Check sheet for the modelled part. Datum: model origin and axes. Units: mm. A direction names the side the tool comes from. Round coordinates to 2 decimals unless told otherwise and drop trailing zeros. Loops run counter-clockwise (first coordinate to the right, second up) from the corner with the lowest first, then second, coordinate; pieces in that order, holes last. Notation, with made-up numbers: (18, 17) - (29, 17) arc R17 cw to (29, 45) - close; hole circle Ø10 at (48, -29.5). An arc over 180 degrees is marked (long way). Put each result on its own line as item: value.
```python
from build123d import *

# Parameters (mm, degrees)
SKETCH1_W           = 44
SKETCH1_H           = 25
SKETCH1_R           = 8.5
SKETCH1_W_2         = 7.5
SKETCH1_H_2         = 4
BOSS_EXTRUDE1_DEPTH = 4
CHAMFER1_SIZE       = 4


with BuildPart() as part:
    # Sketch1 → Boss-Extrude1 (new body)
    with BuildSketch(Plane(origin=(0, 0, 0), x_dir=(1, 0, 0), z_dir=(0, 1, 0))):
        with Locations((22, 12.5)):
            Rectangle(SKETCH1_W, SKETCH1_H)
        with Locations((15, 12.5)):
            Circle(SKETCH1_R, mode=Mode.SUBTRACT)
        with Locations((33.75, 12.5)):
            Rectangle(SKETCH1_W_2, SKETCH1_H_2, mode=Mode.SUBTRACT)
    extrude(amount=BOSS_EXTRUDE1_DEPTH)

    # Chamfer1
    chamfer1_edges = [part.edges().sort_by_distance(p)[0] for p in [
        (0, 2, -25),
        (44, 2, -25),
        (44, 2, 0),
        (0, 2, 0),
    ]]
    chamfer(chamfer1_edges, length=CHAMFER1_SIZE)


solid = part.part
```
Item 1: Section check C-C on y = 0.55. Enter the section's corners in (x, z).
Filled sheet:
outline: (0, -21) - (4, -25) - (40, -25) - (44, -21) - (44, -4) - (40, 0) - (4, 0) - (0, -4) - close; hole circle Ø17 at (15, -12.5); hole (30, -14.5) - (37.5, -14.5) - (37.5, -10.5) - (30, -10.5) - close
Item 2: Go/stop test with a flat-tipped pin: pin 1 (10 mm diameter, centred on x = 15, z = -12.5, fed in from +Y). Record where the tip stops, or that it passes through.
Filled sheet:
pin 1: through
Item 3: Section check B-B on x = 15. Enter the section's corners in (y, z).
Filled sheet:
outline: (0, -25) - (4, -25) - (4, -21) - (0, -21) - close; (0, -4) - (4, -4) - (4, 0) - (0, 0) - close
Item 4: Release check for a two-part mould opening along Z. For faces 1 (the flat face through (42, 2, -23)), 2 (the cylindrical face through (13.16, 1.97, -4.2)), 3 (the flat face through (44, 2, -12)), 4 (the flat face through (37.5, 2, -12)) record: +Z half, -Z half, draft (parallel to the pull), parting line (faces both ways), or undercut.
Filled sheet:
face 1: -Z half
face 2: undercut
face 3: draft
face 4: undercut
Item 5: Section check D-D on z = -16. Enter the section's corners in (x, y), then the cut area to 3 significant figures.
Filled sheet:
outline: (0, 0) - (7.25, 0) - (7.25, 4) - (0, 4) - close; (22.75, 0) - (44, 0) - (44, 4) - (22.75, 4) - close
area: 114 mm²
Item 6: Tool access check on faces 5 (the flat face through (22, 2, -25)), 6 (the flat face through (30, 2, -12)). Record the directions out of +Z, -Z, +X, -X, +Y, -Y that give a thin tool (end or side, any length) a straight path to the whole face; none if there is none.
Filled sheet:
face 5: -Z, +X, -X, +Y, -Y
face 6: +Y, -Y
Item 7: Thickness scan on line 1 (X direction, y = 2.55, z = -12.5); line 2 (Z direction, x = 15, y = 2.55); line 3 (X direction, y = 0.95, z = -15.5). Record the ranges inside material, lowest first. Write a range as from..to.
Filled sheet:
line 1: 0..6.5, 23.5..30, 37.5..44
line 2: -25..-21, -4..0
line 3: 0..7.05, 22.95..44
Item 8: Section check A-A on z = -12.5. Enter the section's corners in (x, y).
Filled sheet:
outline: (0, 0) - (6.5, 0) - (6.5, 4) - (0, 4) - close; (23.5, 0) - (30, 0) - (30, 4) - (23.5, 4) - close; (37.5, 0) - (44, 0) - (44, 4) - (37.5, 4) - close
